CAD build for the part. Positions are in the model's coordinates, mm. Face numbers are marked on the shaded views. A direction names the side the tool comes from. Round coordinates to 2 decimals unless told otherwise and drop trailing zeros. Write each loop counter-clockwise with the first axis right and the second up, starting at its lowest first coordinate (ties: lowest second). Pieces come first, ordered by that corner, then holes. Notation, with made-up numbers: (45, -11) -> (95, -11) arc R20 ccw to (95, 5) -> close; hole circle Ø7 at (-1.5, 43.25). An arc over 180 degrees is marked (long way). Answer in a Markdown table with one row per item. Add a question column.
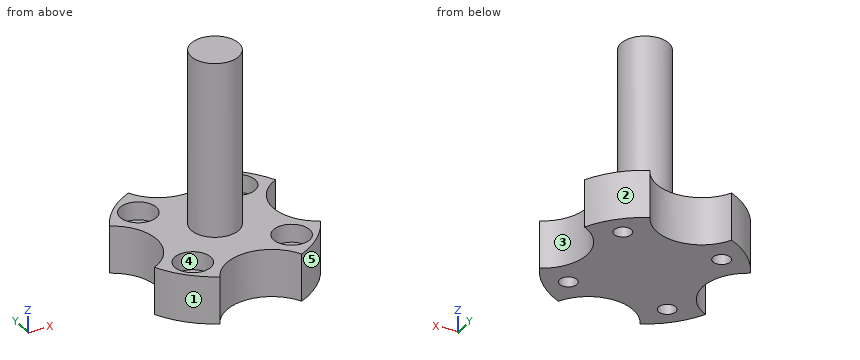
```python
from build123d import *

# Parameters (mm, degrees)
BOSS_EXTRUDE1_DEPTH = 7.874
SKETCH2_R           = 1.4351
CUT_EXTRUDE1_DEPTH  = 7.874
SKETCH3_R           = 3
CUT_EXTRUDE2_DEPTH  = 3
SKETCH4_R           = 3.95
BOSS_EXTRUDE2_DEPTH = 29


with BuildPart() as part:
    # Sketch1 → Boss-Extrude1 (new body)
    with BuildSketch(Plane.XY):
        with BuildLine():
            ThreePointArc((6.727938916, 13.685661765), (0, 9.5), (-6.727938916, 13.685661765))
            ThreePointArc((-6.727938916, 13.685661765), (-10.783378413, 10.783378413), (-13.685661765, 6.727938916))
            ThreePointArc((-13.685661765, 6.727938916), (-9.5, 0), (-13.685661765, -6.727938916))
            ThreePointArc((-13.685661765, -6.727938916), (-10.783378413, -10.783378413), (-6.727938916, -13.685661765))
            ThreePointArc((-6.727938916, -13.685661765), (0, -9.5), (6.727938916, -13.685661765))
            ThreePointArc((6.727938916, -13.685661765), (10.783378413, -10.783378413), (13.685661765, -6.727938916))
            ThreePointArc((13.685661765, -6.727938916), (9.5, 0), (13.685661765, 6.727938916))
            ThreePointArc((13.685661765, 6.727938916), (10.783378413, 10.783378413), (6.727938916, 13.685661765))
        make_face()
    extrude(amount=BOSS_EXTRUDE1_DEPTH)

    # Sketch2 → Cut-Extrude1 (cut)
    with BuildSketch(Plane.XY.offset(7.874)):
        with Locations((-8.131727984, 8.131727984)):
            Circle(SKETCH2_R)
        with Locations((8.131727984, -8.131727984)):
            Circle(SKETCH2_R)
        with Locations((-8.131727984, -8.131727984)):
            Circle(SKETCH2_R)
        with Locations((8.131727984, 8.131727984)):
            Circle(SKETCH2_R)
    extrude(amount=-CUT_EXTRUDE1_DEPTH, mode=Mode.SUBTRACT)

    # Sketch3 → Cut-Extrude2 (cut)
    with BuildSketch(Plane.XY.offset(7.874)):
        with Locations((-8.131727984, 8.131727984)):
            Circle(SKETCH3_R)
        with Locations((-8.131727984, -8.131727984)):
            Circle(SKETCH3_R)
        with Locations((8.131727984, -8.131727984)):
            Circle(SKETCH3_R)
        with Locations((8.131727984, 8.131727984)):
            Circle(SKETCH3_R)
    extrude(amount=-CUT_EXTRUDE2_DEPTH, mode=Mode.SUBTRACT)

    # Sketch4 → Boss-Extrude2 (add)
    with BuildSketch(Plane.XY.offset(7.874)):
        with Locations(Location((0, 0, 0), (0, 0, 180))):
            Circle(SKETCH4_R)
    extrude(amount=BOSS_EXTRUDE2_DEPTH)


solid = part.part
```
Item 1: Pin check, flat tips, straight feed: pin 1 (1.5 mm diameter, centred on x = 2.5, z = 7, fed in from -Y); pin 2 (12 mm diameter, centred on x = -11, y = -1, fed in from -Z); pin 3 (6 mm diameter, centred on y = -9, z = 13.5, fed in from +X); pin 4 (8 mm diameter, centred on x = -8.13, y = 8.13, fed in from +Z). Stop position of each tip, or through.
Item 2: Two-plate mould, pull along Y, no slides. Class the marked faces 1, 2 and 3: +Y half, -Y half, draft (parallel to the pull), parting line (faces both ways), or undercut.
Item 3: Saw through at C-C on z = 6. Give the cut face in (x, y), then the cut area to 3 significant figures.
Item 4: Saw through at D-D on x = -10.5. Give the cut face in (y, z), then the cut area to 3 significant figures.
Item 5: Saw through at A-A on x = 7.75. Give the cut face in (y, z), then the cut area to 3 significant figures.
Item 6: Tool access for the marked faces 4 and 5: list every direction of +Z, -Z, +X, -X, +Y, -Y with a clear straight run to the whole face (end or side of a thin tool).
Item 7: Drill centre lines: probe 1 along X at (y, z) = (-7.5, 2.5); probe 2 along Y at (x, z) = (6, 5); probe 3 along Z at (x, y) = (11, 10). Where is each one in solid material? Low to high.
Item 8: Saw through at B-B on y = 0. Give the cut face in (x, z).
Recorded:
| question | item | result |
|---|---|---|
| 1 | pin 1 | y = -10.24 |
| 1 | pin 2 | z = 0 |
| 1 | pin 3 | through |
| 1 | pin 4 | z = 7.87 |
| 2 | face 1 | -Y half |
| 2 | face 2 | +Y half |
| 2 | face 3 | undercut |
| 3 | outline | (-13.69, -6.73) arc R15.25 ccw to (-6.73, -13.69) arc R7.5 cw to (6.73, -13.69) arc R15.25 ccw to (13.69, -6.73) arc R7.5 cw to (13.69, 6.73) arc R15.25 ccw to (6.73, 13.69) arc R7.5 cw to (-6.73, 13.69) arc R15.25 ccw to (-13.69, 6.73) arc R7.5 cw to start; hole circle Ø6 at (-8.13, -8.13); hole circle Ø6 at (-8.13, 8.13); hole circle Ø6 at (8.13, -8.13); hole circle Ø6 at (8.13, 8.13) |
| 3 | area | 400 mm2 |
| 4 | outline | (-11.06, 0) -> (-3.74, 0) -> (-3.74, 7.87) -> (-6.29, 7.87) -> (-6.29, 4.87) -> (-9.97, 4.87) -> (-9.97, 7.87) -> (-11.06, 7.87) -> close; (3.74, 0) -> (11.06, 0) -> (11.06, 7.87) -> (9.97, 7.87) -> (9.97, 4.87) -> (6.29, 4.87) -> (6.29, 7.87) -> (3.74, 7.87) -> close |
| 4 | area | 93.1 mm2 |
| 5 | outline | (-13.13, 0) -> (-9.52, 0) -> (-9.52, 4.87) -> (-11.11, 4.87) -> (-11.11, 7.87) -> (-13.13, 7.87) -> close; (-6.75, 0) -> (6.75, 0) -> (6.75, 4.87) -> (5.16, 4.87) -> (5.16, 7.87) -> (-5.16, 7.87) -> (-5.16, 4.87) -> (-6.75, 4.87) -> close; (9.52, 0) -> (13.13, 0) -> (13.13, 7.87) -> (11.11, 7.87) -> (11.11, 4.87) -> (9.52, 4.87) -> close |
| 5 | area | 144 mm2 |
| 6 | face 4 | +Z |
| 6 | face 5 | +Z, -Z, +X, -Y |
| 7 | probe 1 | -13.28 to -9.42, -6.84 to 6.84, 9.42 to 13.28 |
| 7 | probe 2 | -12.5 to -10.24, -6.02 to 6.02, 10.24 to 12.5 |
| 7 | probe 3 | 0 to 7.87 |
| 8 | outline | (-9.5, 0) -> (9.5, 0) -> (9.5, 7.87) -> (3.95, 7.87) -> (3.95, 36.87) -> (-3.95, 36.87) -> (-3.95, 7.87) -> (-9.5, 7.87) -> close |
